from build123d import *

# Parameters (mm, degrees)
F0_W     = 228.6
F0_H     = 228.6
F0_W_2   = 25.4
F0_H_2   = 25.4
F1_DEPTH = 114.3
F2_DEPTH = 114.3
F3_W     = 25.4
F3_H     = 25.4
F4_DEPTH = 228.6
F5_W     = 25.4
F5_H     = 25.4
F6_DEPTH = 228.6


with BuildPart() as f1:
    # F0 (on Top) → F1 (new body)
    with BuildSketch(Plane.XY):
        Rectangle(F0_W, F0_H)
        Rectangle(F0_W_2, F0_H_2, mode=Mode.SUBTRACT)
    extrude(amount=F1_DEPTH)

    # F0 (on Top) → F2 (join)
    with BuildSketch(Plane.XY):
        Rectangle(F0_W, F0_H)
        Rectangle(F0_W_2, F0_H_2, mode=Mode.SUBTRACT)
    extrude(amount=-F2_DEPTH)

    # F3 (on face) → F4 (cut)
    with BuildSketch(Plane.XZ.offset(114.3)):
        Rectangle(F3_W, F3_H)
    extrude(amount=-F4_DEPTH, mode=Mode.SUBTRACT)

    # F5 (on face) → F6 (cut)
    with BuildSketch(Plane(origin=(-114.3, 0, 0), x_dir=(0, -1, 0), z_dir=(-1, 0, 0))):
        Rectangle(F5_W, F5_H)
    extrude(amount=-F6_DEPTH, mode=Mode.SUBTRACT)


solid = f1.part
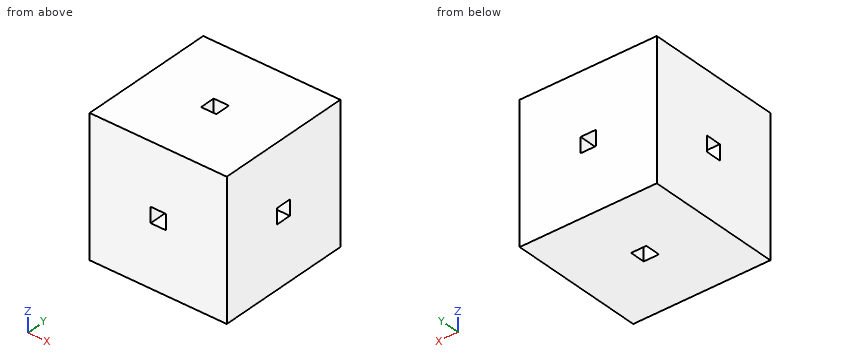
Can you work these out from the model? Positions are in its coordinate system, mm. Round coordinates to 2 decimals unless told otherwise and drop trailing zeros. Order: outer loops, then holes, each group sorted by start corner. A loop starts at its lowest first (then second) coordinate and runs counter-clockwise, first axis right, second up. Notation, with made-up numbers: M -36.75,82.25 L -24.75,82.25 A20 ccw -24.75,107.25 Z; hole C -32,50 d7. An arc over 180 degrees is marked long. Use a Markdown table: item, result.
1) If I drill on line 1 along Y through (x, z) = (74.5, -5), over which ranges is the centre line in solid material (lowest first)?
Geometry says:
| item | result |
|---|---|
| line 1 | y = -114.3 to -12.7, 12.7 to 114.3 |
2) Imagine slicing it at A-A (y = 8.5). List the corners of the cut face in (x, z) for me, then the cut area to 3 significant figures.
Geometry says:
| item | result |
|---|---|
| outline | M -114.3,-114.3 L -12.7,-114.3 L -12.7,-12.7 L -114.3,-12.7 Z; M -114.3,12.7 L -12.7,12.7 L -12.7,114.3 L -114.3,114.3 Z; M 12.7,-114.3 L 114.3,-114.3 L 114.3,-12.7 L 12.7,-12.7 Z; M 12.7,12.7 L 114.3,12.7 L 114.3,114.3 L 12.7,114.3 Z |
| area | 41,300 mm² |
